Here's how the part is built. I have some questions about the finished solid (model axes, mm). Coordinates: 2 decimals unless noted, no trailing zeros. Loops run counter-clockwise (first coordinate to the right, second up) from the corner with the lowest first, then second, coordinate; pieces in that order, holes last. Notation, with made-up numbers: (-32.5, -6) - (-5.5, -6) arc R28 ccw to (-5.5, 25) - close; hole circle Ø1 at (36, 6). An arc over 180 degrees is marked (long way). Use a Markdown table: item, result.
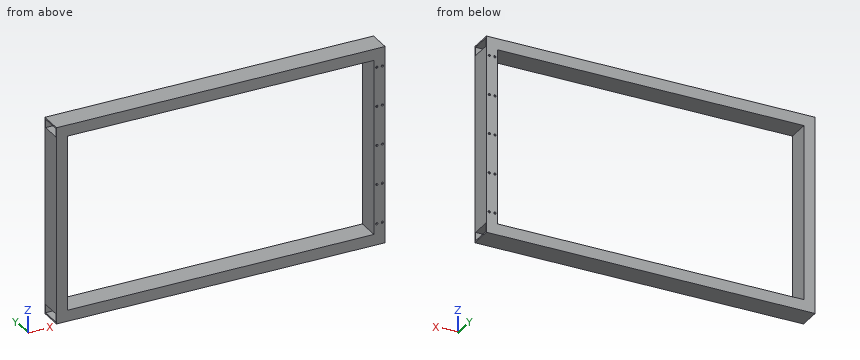
Autodesk Inventor part; units mm, degrees
ref_plane "YZ Plane" through (0, 0, 0) normal (1, 0, 0) x (0, 1, 0)
ref_plane "XZ Plane" through (0, 0, 0) normal (0, 1, 0) x (-1, 0, 0)
ref_plane "XY Plane" through (0, 0, 0) normal (0, 0, 1) x (1, 0, 0)
sketch "Sketch1" plane through (0, 0, 0) normal (1, 0, 0) x (0, 1, 0)
  line L0 (0.0473, 0) -> (50.8473, 0)
  line L1 (50.8473, 0) -> (50.8473, -25.4)
  line L2 (50.8473, -25.4) -> (0.0473, -25.4)
  line L3 (0.0473, -25.4) -> (0.0473, 0)
  line L4 (47.6723, -3.175) -> (3.2223, -3.175)
  line L5 (3.2223, -3.175) -> (3.2223, -22.225)
  line L6 (3.2223, -22.225) -> (47.6723, -22.225)
  line L7 (47.6723, -22.225) -> (47.6723, -3.175)
  dimension "d0" = 25.4
  dimension "d1" = 3.175
  dimension "d2" = 3.175
  dimension "d3" = 3.175
  dimension "d4" = 3.175
  dimension "d5" = 44.45
extrude "Extrusion1" add sketch "Sketch1" along normal blind 750.0112
sketch "Sketch2" plane through (0, 0.0473, 0) normal (0, 0, 1) x (1, 0, 0)
  line L0 (0, 0) -> (0, 50.8)
  line L1 (0, 0) -> (750.0112, 0)
  line L2 (0, 50.8) -> (750.0112, 50.8)
  line L3 (0, 0) -> (25.4, 0)
  line L4 (25.4, 0) -> (25.4, 50.8)
  line L5 (25.4, 50.8) -> (0, 50.8)
  line L6 (0, 50.8) -> (0, 0)
  line L7 (3.175, 47.625) -> (22.225, 47.625)
  line L8 (22.225, 47.625) -> (22.225, 3.175)
  line L9 (22.225, 3.175) -> (3.175, 3.175)
  line L10 (3.175, 3.175) -> (3.175, 47.625)
  dimension "d8" = 25.4
  dimension "d9" = 50.8
  dimension "d10" = 3.175
  dimension "d11" = 3.175
  dimension "d12" = 3.175
  dimension "d13" = 3.175
extrude "Extrusion2" add sketch "Sketch2" along normal blind 399.2118
ref_plane "Work Plane1" through (375.0056, 0, 0) normal (1, 0, 0) x (0, 0, -1)
mirror "Mirror1" about plane through (375.0056, 0, 0) normal (1, 0, 0) of "Extrusion2"
ref_plane "Work Plane2" through (25.4, 0.0473, 199.6059) normal (0, 0, 1) x (1, 0, 0)
mirror "Mirror2" about plane through (25.4, 0.0473, 199.6059) normal (0, 0, 1) of "Extrusion1"
ref_plane "Work Plane3" through (0, 0.0473, -25.4) normal (0, 0, -1) x (-1, 0, 0)
ref_plane "Work Plane4" through (750.0112, 0, 0) normal (1, 0, 0) x (0, 0, -1)
sketch "Sketch5" plane through (0, 50.8473, -25.4) normal (0, 1, 0) x (1, 0, 0)
  line L0 (0, 0) -> (750.0112, 0)
  line L1 (724.6112, -25.4) -> (724.6112, -424.6118)
  point P0 (0, -25.4)
  point P1 (730.9612, -48.4886)
  dimension "d23" = 48.4886
  dimension "d24" = 6.35
hole "Hole1" at (730.9612, 50.8473, 23.0886) direction (0, -1, 0) diameter 5.08 end through all
pattern_linear "Rectangular Pattern1" count 2 spacing 12.7 along (1, 0, 0) count 5 spacing 89.662 along (0, 0, 1) of "Hole1"
properties part number "Resized frame" material "Stainless Steel AISI 440C, Welded"
Q1. I want a section at C-C, the plane x = 368. Write out the boundary of the cut face in (y, z) (3 decimals).
Check values:
| item | result |
|---|---|
| outline | (0.047, -25.4) - (50.847, -25.4) - (50.847, 0) - (0.047, 0) - close; (0.047, 399.212) - (50.847, 399.212) - (50.847, 424.612) - (0.047, 424.612) - close; hole (3.222, -22.225) - (47.672, -22.225) - (47.672, -3.175) - (3.222, -3.175) - close; hole (3.222, 402.387) - (47.672, 402.387) - (47.672, 421.437) - (3.222, 421.437) - close |
Q2. Please list where these lines run through material, in increasing order: L1, parallel to X at y = 4, z = 149 (3 decimals); L2, parallel to Z at x = 321.5, y = 27.5 (3 decimals). Write a range as from..to.
Check values:
| item | result |
|---|---|
| L1 | 0..3.175, 22.225..25.4, 724.611..727.786, 746.836..750.011 |
| L2 | -25.4..-22.225, -3.175..0, 399.212..402.387, 421.437..424.612 |
Q3. I want a section at B-B, the plane y = 15. Write out the boundary of the cut face in (x, z) (3 decimals).
Check values:
| item | result |
|---|---|
| outline | (0, -25.4) - (750.011, -25.4) - (750.011, -22.225) - (0, -22.225) - close; (0, -3.175) - (750.011, -3.175) - (750.011, 402.387) - (0, 402.387) - close; (0, 421.437) - (750.011, 421.437) - (750.011, 424.612) - (0, 424.612) - close; hole (3.175, 0) - (22.225, 0) - (22.225, 399.212) - (3.175, 399.212) - close; hole (25.4, 0) - (724.611, 0) - (724.611, 399.212) - (25.4, 399.212) - close; hole (727.786, 0) - (746.836, 0) - (746.836, 399.212) - (727.786, 399.212) - close |
Q4. I want a section at A-A, the plane z = 130. Write out the boundary of the cut face in (x, y) (3 decimals).
Check values:
| item | result |
|---|---|
| outline | (0, 0.047) - (25.4, 0.047) - (25.4, 50.847) - (0, 50.847) - close; (724.611, 0.047) - (750.011, 0.047) - (750.011, 50.847) - (724.611, 50.847) - close; hole (3.175, 3.222) - (22.225, 3.222) - (22.225, 47.672) - (3.175, 47.672) - close; hole (727.786, 3.222) - (746.836, 3.222) - (746.836, 47.672) - (727.786, 47.672) - close |
